Geometry check sheet. Reference: the model listing, model coordinates, mm. A direction names the side the tool comes from. Round coordinates to 2 decimals unless told otherwise and drop trailing zeros. Order: outer loops, then holes, each group sorted by start corner. A loop starts at its lowest first (then second) coordinate and runs counter-clockwise, first axis right, second up. Notation, with made-up numbers: (69, 2.5) - (103, 2.5) arc R29 cw to (103, 24.5) - close; hole circle Ø7 at (41, -35.5). An arc over 180 degrees is marked (long way). Use a Markdown table: item, result. Add a question column.
(1) Section check D-D on x = 55.5. Record the boundary of the cut face in (y, z).
(2) Gauge pin test, flat ends, axial feed: P1, Ø8, axis at x = 6.5, z = 0, coming from the -Y side; P2, Ø0.9, axis at x = -18.5, z = -0.5, coming from the +Y side; P3, Ø1.5, axis at y = -15.5, z = 15.5, coming from the -X side. Record the tip position at first contact, or that the pin passes through.
(3) Mould release check, pull along Y, two halves, no side actions. Record for faces 5 (the face through (-2, 0, 3)), 6 (the face through (4.62, -15.71, 15.45)), 7 (the face through (62, -18, 0)): released by +Y, released by -Y, zero draft, split by the parting line, or undercut.
(4) Access from +Z, -Z, +X, -X, +Y, -Y to the whole of each face (thin tool, end or side, straight path). Record for faces 1 (the face through (10.341, 18, 17)), 2 (the face through (57, -23, 0)), 3 (the face through (20.481, -16.214, -16.313)), 4 (the face through (20.201, -11.421, 20.687)).
(5) Thickness scan on line 1 along Y through (x, z) = (2, -15); line 2 along Z through (x, y) = (2.75, 15.5). Record the ranges inside material, lowest first. Write a range as [from, to].
(6) Section check A-A on x = 15. Record the boundary of the cut face in (y, z).
(7) Section check B-B on z = 0. Record the boundary of the cut face in (x, y).
(8) Section check C-C on y = 0. Record the boundary of the cut face in (x, z).
```python
from build123d import *

# Parameters (mm, degrees)
ESQUISSE1_W                  = 42
ESQUISSE1_H                  = 42
BOSS_EXTRU_1_DEPTH           = 64
ESQUISSE2_R                  = 11
BOSS_EXTRU_2_DEPTH           = 2
ESQUISSE3_R                  = 2.5
BOSS_EXTRU_3_DEPTH           = 24
TROU_TARAUD_M31_D            = 2.5
TROU_TARAUD_M31_DEPTH        = 4
TROU_TARAUD_M31_TIP          = 0.751075774
ESQUISSE6_OUTSIDE_W          = 65.234
ESQUISSE6_OUTSIDE_H          = 65.234
ESQUISSE6_OUTSIDE_R          = 26
ENL_V_MAT_EXTRU_1_DEPTH      = 71.554943129
ENL_V_MAT_EXTRU_2_DEPTH      = 71.554943129
ENL_V_MAT_EXTRU_2_DEPTH_BACK = 71.554943129
CHANFREIN1_SIZE              = 5
ESQUISSE10_W                 = 26.659419434
ESQUISSE10_H                 = 26.659419434
BOSS_EXTRU_5_DEPTH           = 10
CHANFREIN2_SIZE              = 5
ESQUISSE11_OUTSIDE_W         = 66.102
ESQUISSE11_OUTSIDE_H         = 76.102
ENL_V_MAT_EXTRU_3_DEPTH      = 20
CONG_1_R                     = 4


with BuildPart() as part:
    # Esquisse1 → Boss.-Extru.1 (new body)
    with BuildSketch(Plane(origin=(0, 0, 0), x_dir=(0, 0, -1), z_dir=(1, 0, 0))):
        Rectangle(ESQUISSE1_W, ESQUISSE1_H)
    extrude(amount=BOSS_EXTRU_1_DEPTH)

    # Esquisse2 → Boss.-Extru.2 (add)
    with BuildSketch(Plane(origin=(0, 0, 0), x_dir=(0, 0, -1), z_dir=(1, 0, 0))):
        Circle(ESQUISSE2_R)
    extrude(amount=-BOSS_EXTRU_2_DEPTH)

    # Esquisse3 → Boss.-Extru.3 (add)
    with BuildSketch(Plane.ZY):
        with Locations(Location((0, 0, 0), (0, 0, 180))):
            Circle(ESQUISSE3_R)
    extrude(amount=BOSS_EXTRU_3_DEPTH)

    # Trou taraudé M31
    with Locations(Plane.ZY):
        with Locations((-15.5, 15.5), (15.5, 15.5), (-15.5, -15.5), (15.5, -15.5)):
            Hole(TROU_TARAUD_M31_D / 2, depth=TROU_TARAUD_M31_DEPTH)
            with Locations((0, 0, -(TROU_TARAUD_M31_DEPTH + TROU_TARAUD_M31_TIP / 2))):  # 118° drill point
                Cone(0, TROU_TARAUD_M31_D / 2, TROU_TARAUD_M31_TIP, mode=Mode.SUBTRACT)

    # Esquisse6 outside → Enlèv. mat.-Extru.1 (cut, through all)
    with BuildSketch(Plane(origin=(0, 0, 0), x_dir=(0, 0, -1), z_dir=(1, 0, 0))):
        Rectangle(ESQUISSE6_OUTSIDE_W, ESQUISSE6_OUTSIDE_H)
        Circle(ESQUISSE6_OUTSIDE_R, mode=Mode.SUBTRACT)
    extrude(amount=ENL_V_MAT_EXTRU_1_DEPTH, mode=Mode.SUBTRACT)

    # Esquisse7 → Enlèv. mat.-Extru.2 (cut, two sides: drawn at the far end of the back side and taken through both)
    with BuildSketch(Plane.XY.offset(-ENL_V_MAT_EXTRU_2_DEPTH_BACK)):
        Polygon((-215.91206667, 2), (-24, 2), (-9, 2), (-9, 2.5), (-9, 194.41206667), (-270.377319091, 475.486545052), (-477.289385761, 283.074478383), align=None)
    extrude(amount=ENL_V_MAT_EXTRU_2_DEPTH + ENL_V_MAT_EXTRU_2_DEPTH_BACK, mode=Mode.SUBTRACT)

    # Chanfrein1
    chanfrein1_edges = [part.edges().sort_by_distance(p)[0] for p in [
        (64, 0, 21),
        (64, -21, 0),
        (64, 0, -21),
        (64, 21, 0),
        (64, -18.384776311, 18.384776311),
        (64, 18.384776311, 18.384776311),
        (64, -18.384776311, -18.384776311),
        (64, 18.384776311, -18.384776311),
    ]]
    chamfer(chanfrein1_edges, length=CHANFREIN1_SIZE)

    # Esquisse10 → Boss.-Extru.5 (add)
    with BuildSketch(Plane.XZ.offset(21)):
        with Locations((43.670290283, 0)):
            Rectangle(ESQUISSE10_W, ESQUISSE10_H)
    extrude(amount=BOSS_EXTRU_5_DEPTH)

    # Chanfrein2
    chanfrein2_edges = [part.edges().sort_by_distance(p)[0] for p in [
        (57, -31, 0),
        (43.670290283, -31, 13.329709717),
        (43.670290283, -31, -13.329709717),
    ]]
    chamfer(chanfrein2_edges, length=CHANFREIN2_SIZE)

    # Esquisse11 outside → Enlèv. mat.-Extru.3 (cut)
    with BuildSketch(Plane.ZY.offset(-30.340580566)):
        with Locations((0, -5)):
            Rectangle(ESQUISSE11_OUTSIDE_W, ESQUISSE11_OUTSIDE_H)
        Polygon((0, 32.526911935), (-32.526911935, 0), (0, -32.526911935), (32.526911935, 0), align=None, mode=Mode.SUBTRACT)
    extrude(amount=ENL_V_MAT_EXTRU_3_DEPTH, mode=Mode.SUBTRACT)

    # Congé1
    cong_1_edges = [part.edges().sort_by_distance(p)[0] for p in [
        (20.340580566, 21, -11.526911935),
        (20.340580566, 21, 11.526911935),
        (20.340580566, 11.526911935, 21),
        (20.340580566, 11.526911935, -21),
        (20.340580566, -21, -11.526911935),
        (20.340580566, -11.526911935, -21),
        (20.340580566, -21, 11.526911935),
        (20.340580566, -11.526911935, 21),
    ]]
    fillet(cong_1_edges, radius=CONG_1_R)


solid = part.part
```
Check sheet entries:
| question | item | result |
|---|---|---|
| 1 | outline | (-27.5, -11.83) - (-26, -13.33) - (-21, -13.33) - (-21, -15.33) arc R26 ccw to (-15.33, -21) - (15.33, -21) arc R26 ccw to (21, -15.33) - (21, 15.33) arc R26 ccw to (15.33, 21) - (-15.33, 21) arc R26 ccw to (-21, 15.33) - (-21, 13.33) - (-26, 13.33) - (-27.5, 11.83) - close |
| 2 | P1 | stops at y = -21 |
| 2 | P2 | stops at y = 2 |
| 2 | P3 | stops at x = 4.3 |
| 3 | face 5 | zero draft |
| 3 | face 6 | undercut |
| 3 | face 7 | released by -Y |
| 4 | face 1 | +Z, +Y |
| 4 | face 2 | +Z, -Z, +X, -Y |
| 4 | face 3 | -Z, -Y |
| 4 | face 4 | +Z, -Y |
| 5 | line 1 | y = [-21, -16.65], [-14.35, 14.35], [16.65, 21] |
| 5 | line 2 | z = [-20.87, -16.75], [-14.25, 14.25], [16.75, 20.87] |
| 6 | outline | (-21, -9.87) arc R4 ccw to (-19.83, -12.7) - (-12.7, -19.83) arc R4 ccw to (-9.87, -21) - (9.87, -21) arc R4 ccw to (12.7, -19.83) - (19.83, -12.7) arc R4 ccw to (21, -9.87) - (21, 9.87) arc R4 ccw to (19.83, 12.7) - (12.7, 19.83) arc R4 ccw to (9.87, 21) - (-9.87, 21) arc R4 ccw to (-12.7, 19.83) - (-19.83, 12.7) arc R4 ccw to (-21, 9.87) - close |
| 7 | outline | (-24, -2.5) - (-2, -2.5) - (-2, -11) - (0, -11) - (0, -21) - (30.34, -21) - (30.34, -31) - (52, -31) - (57, -26) - (57, -21) - (59, -21) - (64, -16) - (64, 16) - (59, 21) - (0, 21) - (0, 11) - (-2, 11) - (-2, 2.5) - (-9, 2.5) - (-9, 2) - (-24, 2) - close |
| 8 | outline | (-24, -2.5) - (-2, -2.5) - (-2, -11) - (0, -11) - (0, -21) - (59, -21) - (64, -16) - (64, 16) - (59, 21) - (0, 21) - (0, 11) - (-2, 11) - (-2, 2.5) - (-24, 2.5) - close |
